```python
from build123d import *

# Parameters (mm, degrees)
BOSS_EXTRUDE1_DEPTH = 30
CUT_EXTRUDE1_DEPTH  = 82
SKETCH3_R           = 2.25
CUT_EXTRUDE2_DEPTH  = 60
HOLE2_D             = 4.5
HOLE2_CBORE_D       = 6
HOLE2_CBORE_DEPTH   = 10


with BuildPart() as part:
    # Sketch1 → Boss-Extrude1 (new body, symmetric)
    with BuildSketch(Plane.XY):
        with BuildLine():
            Line((17, -28), (17, -21.840329668))
            ThreePointArc((17, -21.840329668), (17.377125597, -19.935327763), (18.451612903, -18.31769585))
            ThreePointArc((18.451612903, -18.31769585), (19.07334688, -17.669392712), (19.672315573, -17))
            Line((19.672315573, -17), (67, -17))
            Line((67, -17), (67, -20))
            Line((67, -20), (29, -20))
            Line((29, -20), (29, -23))
            Line((29, -23), (69, -23))
            Line((69, -23), (69, -26))
            Line((69, -26), (29, -35))
            Line((29, -35), (-13, -35))
            Line((-13, -35), (-13, -32))
            Line((-13, -32), (13, -32))
            ThreePointArc((13, -32), (15.828427125, -30.828427125), (17, -28))
        make_face()
    extrude(amount=BOSS_EXTRUDE1_DEPTH, both=True)

    # Sketch2 → Cut-Extrude1 (cut)
    with BuildSketch(Plane(origin=(69, 0, 0), x_dir=(0, 0, -1), z_dir=(1, 0, 0))):
        with BuildLine():
            Line((-22.937838499, -22.36116349), (-22.937838499, -22.406895186))
            ThreePointArc((-22.937838499, -22.406895186), (-22.880874155, -22.988738058), (-22.712144413, -23.548484732))
            Line((-22.712144413, -23.548484732), (-18, -35))
            Line((-18, -35), (-30, -35))
            Line((-30, -35), (-30, -17))
            Line((-30, -17), (-25, -17))
            ThreePointArc((-25, -17), (-24.666676832, -18.795028508), (-23.711149062, -20.350727181))
            ThreePointArc((-23.711149062, -20.350727181), (-23.1378324, -21.284146385), (-22.937838499, -22.36116349))
        make_face()
        with BuildLine():
            Line((30, -35), (18, -35))
            Line((18, -35), (22.712144413, -23.548484732))
            ThreePointArc((22.712144413, -23.548484732), (22.880874155, -22.988738058), (22.937838499, -22.406895186))
            Line((22.937838499, -22.406895186), (22.937838499, -22.36116349))
            ThreePointArc((22.937838499, -22.36116349), (23.1378324, -21.284146385), (23.711149062, -20.350727181))
            ThreePointArc((23.711149062, -20.350727181), (24.666676832, -18.795028508), (25, -17))
            Line((25, -17), (30, -17))
            Line((30, -17), (30, -35))
        make_face()
    extrude(amount=-CUT_EXTRUDE1_DEPTH, mode=Mode.SUBTRACT)

    # Sketch3 → Cut-Extrude2 (cut)
    with BuildSketch(Plane(origin=(0, -35, 0), x_dir=(-1, 0, 0), z_dir=(0, -1, 0))):
        with Locations((3, -10)):
            Circle(SKETCH3_R)
        with Locations((3, 10)):
            Circle(SKETCH3_R)
    extrude(amount=-CUT_EXTRUDE2_DEPTH, mode=Mode.SUBTRACT)

    # Hole2 (through all)
    with Locations(Plane(origin=(0, -35, 0), x_dir=(-1, 0, 0), z_dir=(0, -1, 0))):
        with Locations((-63, 8), (-63, -8), (-43, 0)):
            CounterBoreHole(HOLE2_D / 2, HOLE2_CBORE_D / 2, HOLE2_CBORE_DEPTH)


solid = part.part
```
Could you check a few things on this model? Use its own coordinates, in mm. A direction names the side the tool comes from. Round coordinates to 2 decimals unless told otherwise and drop trailing zeros. Loops run counter-clockwise (first coordinate to the right, second up) from the corner with the lowest first, then second, coordinate; pieces in that order, holes last. Notation, with made-up numbers: (64.5, -8) - (98.5, -8) arc R10 ccw to (98.5, -4) - close; hole circle Ø4 at (-38, 6). An arc over 180 degrees is marked (long way). Use CSV: the item, a comma, the result in double quotes.
Item 1: If we section it at B-B on z = -17: List the corners of the cut face in (x, y) for me, then the cut area to 3 significant figures.
Here are the results:
outline,"(-13, -35) - (29, -35) - (69, -26) - (69, -23) - (29, -23) - (29, -20) - (67, -20) - (67, -17) - (19.67, -17) arc R26 cw to (18.45, -18.32) arc R5 ccw to (17, -21.84) - (17, -28) arc R4 cw to (13, -32) - (-13, -32) - close"
area,"719 mm²"
Item 2: If we section it at A-A on x = -3: List the corners of the cut face in (y, z) for me.
Here are the results:
outline,"(-35, -18) - (-32, -19.23) - (-32, -12.25) - (-35, -12.25) - close; (-35, -7.75) - (-32, -7.75) - (-32, 7.75) - (-35, 7.75) - close; (-35, 12.25) - (-32, 12.25) - (-32, 19.23) - (-35, 18) - close"
Item 3: If we section it at D-D on x = 48: List the corners of the cut face in (y, z) for me (3 decimals), then the cut area to 3 significant figures.
Here are the results:
outline,"(-30.725, -19.759) - (-23.548, -22.712) arc R3 ccw to (-23, -22.879) - (-23, 22.879) arc R3 ccw to (-23.548, 22.712) - (-30.725, 19.759) - close; (-20, -24) arc R5 ccw to (-17, -25) - (-17, 25) arc R5 ccw to (-20, 24) - close"
area,"478 mm²"
Item 4: If we mould it in two halves opening along Y, with no side actions, what happens to faces 1 (the flat face through (48, -20, 0)), 2 (the cylindrical face through (42.462, -18.819, -24.657)), 3 (the cylindrical face through (60.752, -18.479, 7.901))? For each: pulls with the +Y half, pulls with the -Y half, needs draft (parallel to the pull), parting line crosses it, or undercut.
Here are the results:
face 1,"undercut"
face 2,"pulls with the -Y half"
face 3,"needs draft"
Item 5: I need wall thicknesses on L1, parallel to Y at x = 60, z = 7 (3 decimals); L2, parallel to Y at x = 40, z = -15.5 (3 decimals); L3, parallel to X at y = -25.7, z = 8. Which ranges of each line are inside material? Lowest first, please. Write a range as [from, to].
Here are the results:
L1,"y = [-28.025, -23], [-20, -17]"
L2,"y = [-32.525, -23], [-20, -17]"
L3,"x = [17, 60], [66, 69]"
Item 6: If we section it at C-C on x = 28: List the corners of the cut face in (y, z) for me.
Here are the results:
outline,"(-35, -18) - (-23.55, -22.71) arc R3 ccw to (-22.41, -22.94) - (-22.36, -22.94) arc R3 cw to (-20.35, -23.71) arc R5 ccw to (-17, -25) - (-17, 25) arc R5 ccw to (-20.35, 23.71) arc R3 cw to (-22.36, 22.94) - (-22.41, 22.94) arc R3 ccw to (-23.55, 22.71) - (-35, 18) - close"
Item 7: For faces 4 (the flat face through (67, -18, 0)), 5 (the cylindrical face through (40.14, -28.82, -0.9)), 6 (the flat face through (49, -23, 0)), which set-ups out of +Z, -Z, +X, -X, +Y, -Y let a thin tool reach every point of the face, with its end or its side?
Here are the results:
face 4,"+Z, -Z, +X, +Y"
face 5,"-Y"
face 6,"+Z, -Z, +X"
Item 8: Will these pins go through, and if not, where does the flat tip stop? pin 1 (13 mm diameter, centred on x = 4.5, z = -0.5, fed in from +Y); pin 2 (4 mm diameter, centred on x = -3, z = -10, fed in from +Y); pin 3 (5 mm diameter, centred on x = 43, z = 1, fed in from -Y); pin 4 (10 mm diameter, centred on x = 48, y = -24, fed in from -Z).
Here are the results:
pin 1,"stops at y = -32"
pin 2,"passes through"
pin 3,"stops at y = -32.38"
pin 4,"stops at z = -24.58"
